```python
from build123d import *

# Parameters (mm, degrees)
F0_W      = 266.7
F0_H      = 127
F1_DEPTH  = 12.7
F2_W      = 241.3
F2_H      = 50.8
F3_DEPTH  = 101.6
F4_W      = 266.7
F4_H      = 12.7
F5_DEPTH  = 50.8
F6_W      = 241.3
F6_H      = 19.05
F7_DEPTH  = 63.5
F8_W      = 50.8
F8_H      = 25.4
F9_DEPTH  = 63.5
F10_W     = 31.75
F10_H     = 44.45
F11_DEPTH = 6.35
F12_W     = 241.3
F12_H     = 12.7
F13_DEPTH = 63.5
F14_W     = 31.75
F14_H     = 6.35
F15_DEPTH = 6.35
F16_W     = 25.4
F16_H     = 12.7
F17_DEPTH = 12.7


with BuildPart() as f1:
    # F0 (on Top) → F1 (new body)
    with BuildSketch(Plane.XY):
        with Locations((133.35, 63.5)):
            Rectangle(F0_W, F0_H)
    extrude(amount=F1_DEPTH)

    # F2 (on face) → F3 (join)
    with BuildSketch(Plane.XY.offset(12.7)):
        Polygon((0, 63.5), (0, 50.8), (266.7, 50.8), (266.7, 63.5), (266.7, 114.3), (266.7, 127), (0, 127), (0, 114.3), align=None)
        with Locations((133.35, 88.9)):
            Rectangle(F2_W, F2_H, mode=Mode.SUBTRACT)
    extrude(amount=F3_DEPTH)

    # F4 (on face) → F5 (join, through all)
    with BuildSketch(Plane.XZ.offset(-50.8)):
        with Locations((133.35, 88.9)):
            Rectangle(F4_W, F4_H)
    extrude(amount=F5_DEPTH)

    # F6 (on face) → F7 (cut, through all)
    with BuildSketch(Plane(origin=(0, 127, 0), x_dir=(-1, 0, 0), z_dir=(0, 1, 0))):
        with Locations((-133.35, 22.225)):
            Rectangle(F6_W, F6_H)
    extrude(amount=-F7_DEPTH, mode=Mode.SUBTRACT)

    # F8 (on face) → F9 (cut, through all)
    with BuildSketch(Plane.XZ.offset(-50.8)):
        with Locations((133.35, 25.4)):
            Rectangle(F8_W, F8_H)
    extrude(amount=-F9_DEPTH, mode=Mode.SUBTRACT)

    # F10 (on face) → F11 (cut)
    with BuildSketch(Plane.XY.offset(95.25)):
        with Locations((133.35, 28.575)):
            Rectangle(F10_W, F10_H)
    extrude(amount=-F11_DEPTH, mode=Mode.SUBTRACT)

    # F12 (on face) → F13 (join, through all)
    with BuildSketch(Plane(origin=(0, 127, 0), x_dir=(-1, 0, 0), z_dir=(0, 1, 0))):
        with Locations((-133.35, 38.1)):
            Rectangle(F12_W, F12_H)
    extrude(amount=-F13_DEPTH)

    # F14 (on face) → F15 (cut, through all)
    with BuildSketch(Plane.XY.offset(88.9)):
        with Locations((133.35, 47.625)):
            Rectangle(F14_W, F14_H)
    extrude(amount=-F15_DEPTH, mode=Mode.SUBTRACT)

    # F16 (on face) → F17 (cut, through all)
    with BuildSketch(Plane.XY.offset(44.45)):
        with Locations((215.9, 69.85)):
            Rectangle(F16_W, F16_H)
        with Locations((50.8, 69.85)):
            Rectangle(F16_W, F16_H)
        with Locations((133.35, 69.85)):
            Rectangle(F16_W, F16_H)
    extrude(amount=-F17_DEPTH, mode=Mode.SUBTRACT)


solid = f1.part
```
Design review of the part built by this model. Coordinates are the model's own, in mm. A direction names the side the tool comes from. Round coordinates to 2 decimals unless told otherwise and drop trailing zeros. Order: outer loops, then holes, each group sorted by start corner. A loop starts at its lowest first (then second) coordinate and runs counter-clockwise, first axis right, second up. Notation, with made-up numbers: (-27, -36) - (21, -36) arc R26 ccw to (21, -8) - close; hole circle Ø6 at (27.25, 61.5). An arc over 180 degrees is marked (long way). Return JSON: item names as keys, results as strings.
Q1. Consider section A-A on x = 136.5. Write out the cut boundary in (y, z), plus the area to 3 significant figures.
Computed values:
{"outline": "(0, 0) - (127, 0) - (127, 12.7) - (0, 12.7) - close; (0, 82.55) - (44.45, 82.55) - (44.45, 88.9) - (6.35, 88.9) - (6.35, 95.25) - (0, 95.25) - close; (50.8, 38.1) - (63.5, 38.1) - (63.5, 114.3) - (50.8, 114.3) - close; (76.2, 31.75) - (127, 31.75) - (127, 114.3) - (114.3, 114.3) - (114.3, 44.45) - (76.2, 44.45) - close", "area": "4,440 mm2"}
Q2. Consider section D-D on x = 222.5. Write out the cut boundary in (y, z).
Computed values:
{"outline": "(0, 0) - (127, 0) - (127, 12.7) - (63.5, 12.7) - (63.5, 114.3) - (50.8, 114.3) - (50.8, 95.25) - (0, 95.25) - (0, 82.55) - (50.8, 82.55) - (50.8, 12.7) - (0, 12.7) - close; (76.2, 31.75) - (127, 31.75) - (127, 114.3) - (114.3, 114.3) - (114.3, 44.45) - (76.2, 44.45) - close"}
Q3. Consider section C-C on y = 86. Write out the cut boundary in (x, z), plus the area to 3 significant figures.
Computed values:
{"outline": "(0, 0) - (266.7, 0) - (266.7, 114.3) - (254, 114.3) - (254, 44.45) - (12.7, 44.45) - (12.7, 114.3) - (0, 114.3) - close; hole (12.7, 12.7) - (254, 12.7) - (254, 31.75) - (12.7, 31.75) - close", "area": "9,030 mm2"}
Q4. Consider section B-B on y = 10.5. Write out the cut boundary in (x, z) (3 decimals).
Computed values:
{"outline": "(0, 0) - (266.7, 0) - (266.7, 12.7) - (0, 12.7) - close; (0, 82.55) - (266.7, 82.55) - (266.7, 95.25) - (149.225, 95.25) - (149.225, 88.9) - (117.475, 88.9) - (117.475, 95.25) - (0, 95.25) - close"}
Q5. Wall thickness on L1, parallel to Y at x = 119.5, z = 85; L2, parallel to Z at x = 130, y = 77.5; L3, parallel to Z at x = 84, y = 23.5: over which ranges is each line inside the solid? List them lowest first. Write a range as [from, to].
Computed values:
{"L1": "y = [0, 44.45], [50.8, 63.5], [114.3, 127]", "L2": "z = [0, 12.7], [31.75, 44.45]", "L3": "z = [0, 12.7], [82.55, 95.25]"}
Q6. The part is to be moulded in two halves that separate along Y. For faces 1 (the flat face through (107.95, 57, 25)), 2 (the flat face through (114, 63.5, 35)), 3 (the flat face through (132, 114.3, 79)), say which applies: pulls with the +Y half, pulls with the -Y half, needs draft (parallel to the pull), parting line crosses it, or undercut.
Computed values:
{"face 1": "needs draft", "face 2": "pulls with the -Y half", "face 3": "undercut"}
Q7. For pin 1 Ø14 at (x, z) = (45, 37.5) entering from -Y; pin 2 Ø12 at (x, y) = (205, 19) entering from +Z, all flat-tipped, find the tip position at first contact; note any pin that passes through.
Computed values:
{"pin 1": "stops at y = 50.8", "pin 2": "stops at z = 95.25"}
Q8. Machinability: for faces 4 (the flat face through (133, 57, 38.1)), 5 (the flat face through (131, 3, 95.25)), 6 (the flat face through (132, 63.5, 63)), 7 (the flat face through (12.7, 95, 22)), 8 (the flat face through (117.475, 28, 92)), which of the approach directions +Z, -Z, +X, -X, +Y, -Y give a long, thin tool a straight path to every point of the face, cutting with its end or side? Answer none if there is none.
Computed values:
{"face 4": "-Y", "face 5": "+Z, +X, -X, -Y", "face 6": "none", "face 7": "+Y", "face 8": "+Z"}
